from build123d import *

# Parameters (mm, degrees)
SKETCH_1_R               = 36
EXTRUDE_1_DEPTH          = 90
SKETCH_2_W               = 22
SKETCH_2_H               = 6.721726998
CUT_EXTRUDE_1_DEPTH      = 60
CUT_EXTRUDE_2_DEPTH      = 108.060730429
CUT_EXTRUDE_2_DEPTH_BACK = 108.060730429
EXTRUDE_3_DEPTH          = 20
SKETCH_5_R               = 2.1
CUT_EXTRUDE_3_DEPTH      = 126.87569265
PATTERN_LINEAR_1_COUNT   = 2
PATTERN_LINEAR_1_PITCH   = 60
EXTRUDE_4_DEPTH          = 20


with BuildPart() as part:
    # 草圖1 → 填料-伸長1 (new body)
    with BuildSketch(Plane.XY):
        with BuildLine():
            Line((-41, 0), (-41, -41))
            Line((-41, -41), (41, -41))
            Line((41, -41), (41, 0))
            ThreePointArc((41, 0), (0, 41), (-41, 0))
        make_face()
        with Locations(Location((0, 0, 0), (0, 0, 180))):
            Circle(SKETCH_1_R, mode=Mode.SUBTRACT)
    extrude(amount=EXTRUDE_1_DEPTH)

    # 草圖2 → 除料-伸長1 (cut)
    with BuildSketch(Plane.XY):
        with Locations((0, -37.639136501)):
            Rectangle(SKETCH_2_W, SKETCH_2_H)
    extrude(amount=CUT_EXTRUDE_1_DEPTH, mode=Mode.SUBTRACT)

    # 草圖3 → 除料-伸長2 (cut, two sides: drawn at the far end of the back side and taken through both)
    with BuildSketch(Plane(origin=(0, 0, 0), x_dir=(0, 0, -1), z_dir=(1, 0, 0)).offset(-CUT_EXTRUDE_2_DEPTH_BACK)):
        Polygon((0, 41), (-90, 41), (-90, -21), (-45, -21), (-45, 0), (0, 0), align=None)
    extrude(amount=CUT_EXTRUDE_2_DEPTH + CUT_EXTRUDE_2_DEPTH_BACK, mode=Mode.SUBTRACT)

    # 草圖4 → 填料-伸長3 (add)
    with BuildSketch(Plane.XY.offset(90)):
        with BuildLine():
            Line((-30, -73.7), (-30, -27.946386022))
            ThreePointArc((-30, -27.946386022), (-32.791276328, -24.611637258), (-35.213640705, -21))
            Line((-35.213640705, -21), (-41, -21))
            Line((-41, -21), (-41, -68.7))
            Line((-41, -68.7), (-55, -68.7))
            Line((-55, -68.7), (-55, -73.7))
            Line((-55, -73.7), (-30, -73.7))
        make_face()
        with BuildLine():
            Line((30, -73.7), (30, -27.946386022))
            ThreePointArc((30, -27.946386022), (32.791276328, -24.611637258), (35.213640705, -21))
            Line((35.213640705, -21), (41, -21))
            Line((41, -21), (41, -68.7))
            Line((41, -68.7), (55, -68.7))
            Line((55, -68.7), (55, -73.7))
            Line((55, -73.7), (30, -73.7))
        make_face()
    extrude_3 = extrude(amount=-EXTRUDE_3_DEPTH)

    # 草圖5 → 除料-伸長3 (cut, through all)
    with BuildSketch(Plane(origin=(0, -68.7, 0), x_dir=(1, 0, 0), z_dir=(0, 1, 0))):
        with Locations(Location((-48, -80, 0), (0, 0, 180))):
            Circle(SKETCH_5_R)
        with Locations(Location((48, -80, 0), (0, 0, 180))):
            Circle(SKETCH_5_R)
        with BuildLine():
            Line((45, -70), (45, -66.851466146))
            Line((45, -66.851466146), (57.675759509, -66.851466146))
            Line((57.675759509, -66.851466146), (57.675759509, -92.046945096))
            Line((57.675759509, -92.046945096), (45, -92.046945096))
            Line((45, -92.046945096), (45, -90))
            ThreePointArc((45, -90), (55, -80), (45, -70))
        make_face()
        with BuildLine():
            Line((-57.675759509, -92.046945096), (-45, -92.046945096))
            Line((-45, -92.046945096), (-45, -90))
            ThreePointArc((-45, -90), (-55, -80), (-45, -70))
            Line((-45, -70), (-45, -66.851466146))
            Line((-45, -66.851466146), (-57.675759509, -66.851466146))
            Line((-57.675759509, -66.851466146), (-57.675759509, -92.046945096))
        make_face()
    cut_extrude_3 = extrude(amount=-CUT_EXTRUDE_3_DEPTH, mode=Mode.SUBTRACT)

    # 直線複製排列1: 填料-伸長3, 除料-伸長3 ×2
    with Locations(*[(0, 0, -i * PATTERN_LINEAR_1_PITCH) for i in range(1, PATTERN_LINEAR_1_COUNT)]):
        add(extrude_3)
        add(cut_extrude_3, mode=Mode.SUBTRACT)

    # 草圖6 → 填料-伸長4 (add)
    with BuildSketch(Plane.XY.offset(90)):
        with BuildLine():
            Line((-29.240383034, -21), (-41.000001526, -21))
            Line((-41.000001526, -21), (-41, -41))
            Line((-41, -41), (41, -41))
            Line((41, -41), (41, -21))
            Line((41, -21), (29.240383034, -21))
            ThreePointArc((29.240383034, -21), (0, -36), (-29.240383034, -21))
        make_face()
    extrude(amount=EXTRUDE_4_DEPTH)


solid = part.part
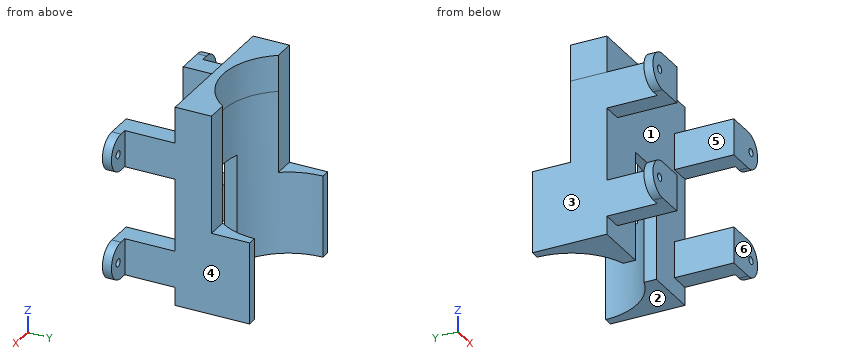
Work out the finished part from the listing and answer in its coordinate system (mm). Face numbers are marked on the shaded views. A direction names the side the tool comes from. Give positions to 0.01 mm unless a question says otherwise; leave off trailing zeros. Write each loop counter-clockwise with the first axis right and the second up, starting at its lowest first coordinate (ties: lowest second). Pieces come first, ordered by that corner, then holes.
Q1. A tool of negligible diameter and unlimited length cuts with its end or side. For the marked faces 4, 5 and 6, from which of +Z, -Z, +X, -X, +Y, -Y can it reach the whole face along a straight path? Write none if from no direction.
Answer:
face 4: +Z, -Z, +X, +Y
face 5: +Z, -Z, -Y
face 6: +Z, -Z, +X, -X, -Y
Q2. The part is cut by section C-C on z = 20. Give the vertices of the cut face in (x, y).
Answer:
outline: (-55, -73.7) - (-50.1, -73.7) - (-50.1, -68.7) - (-55, -68.7) - close; (-45.9, -73.7) - (-30, -73.7) - (-30, -41) - (-11, -41) - (-11, -34.28) arc R36 cw to (-36, 0) - (-41, 0) - (-41, -68.7) - (-45.9, -68.7) - close; (11, -41) - (30, -41) - (30, -73.7) - (45.9, -73.7) - (45.9, -68.7) - (41, -68.7) - (41, 0) - (36, 0) arc R36 cw to (11, -34.28) - close; (50.1, -73.7) - (55, -73.7) - (55, -68.7) - (50.1, -68.7) - close
Q3. For a pull along X with two mould halves and no side action, classify the marked faces 1, 2 and 3 as released by +X, released by -X, zero draft, split by the parting line, or undercut.
Answer:
face 1: undercut
face 2: zero draft
face 3: released by -X
Q4. Given pin 1 (3.5 mm diameter, centred on y = -36.5, z = 36.5, fed in from -X); pin 2 (11 mm diameter, centred on x = -48.5, z = 20.5, fed in from +Y); pin 3 (12 mm diameter, centred on x = 35.5, y = -54, fed in from +Z), each flat-ended and moving along its own axis, determine where each tip first touches the part or whether it passes through.
Answer:
pin 1: stops at x = -41
pin 2: stops at y = -68.7
pin 3: stops at z = 90
Q5. The part is cut by section D-D on x = 48. Give the vertices of the cut face in (y, z), and give its area (3 significant figures).
Answer:
outline: (-73.7, 10.46) - (-68.7, 10.46) - (-68.7, 17.9) - (-73.7, 17.9) - close; (-73.7, 22.1) - (-68.7, 22.1) - (-68.7, 29.54) - (-73.7, 29.54) - close; (-73.7, 70.46) - (-68.7, 70.46) - (-68.7, 77.9) - (-73.7, 77.9) - close; (-73.7, 82.1) - (-68.7, 82.1) - (-68.7, 89.54) - (-73.7, 89.54) - close
area: 149 mm2
Q6. The part is cut by section B-B on y = -63. Give the vertices of the cut face in (x, z).
Answer:
outline: (-41, 10) - (-30, 10) - (-30, 30) - (-41, 30) - close; (-41, 70) - (-30, 70) - (-30, 90) - (-41, 90) - close; (30, 10) - (41, 10) - (41, 30) - (30, 30) - close; (30, 70) - (41, 70) - (41, 90) - (30, 90) - close
Q7. Straight lines are drawn through the part: L1, parallel to Z at x = -48, y = -69.65; L2, parallel to X at y = -38, z = 53; L3, parallel to X at y = -47.5, z = 83. For each, find the intervals that lie inside material, in ascending order.
Answer:
L1: z = 10.46 to 17.9, 22.1 to 29.54, 70.46 to 77.9, 82.1 to 89.54
L2: x = -41 to -11, 11 to 41
L3: x = -41 to -30, 30 to 41
Q8. The part is cut by section A-A on z = 33. Give the vertices of the cut face in (x, y).
Answer:
outline: (-41, -41) - (-11, -41) - (-11, -34.28) arc R36 cw to (-36, 0) - (-41, 0) - close; (11, -41) - (41, -41) - (41, 0) - (36, 0) arc R36 cw to (11, -34.28) - close
